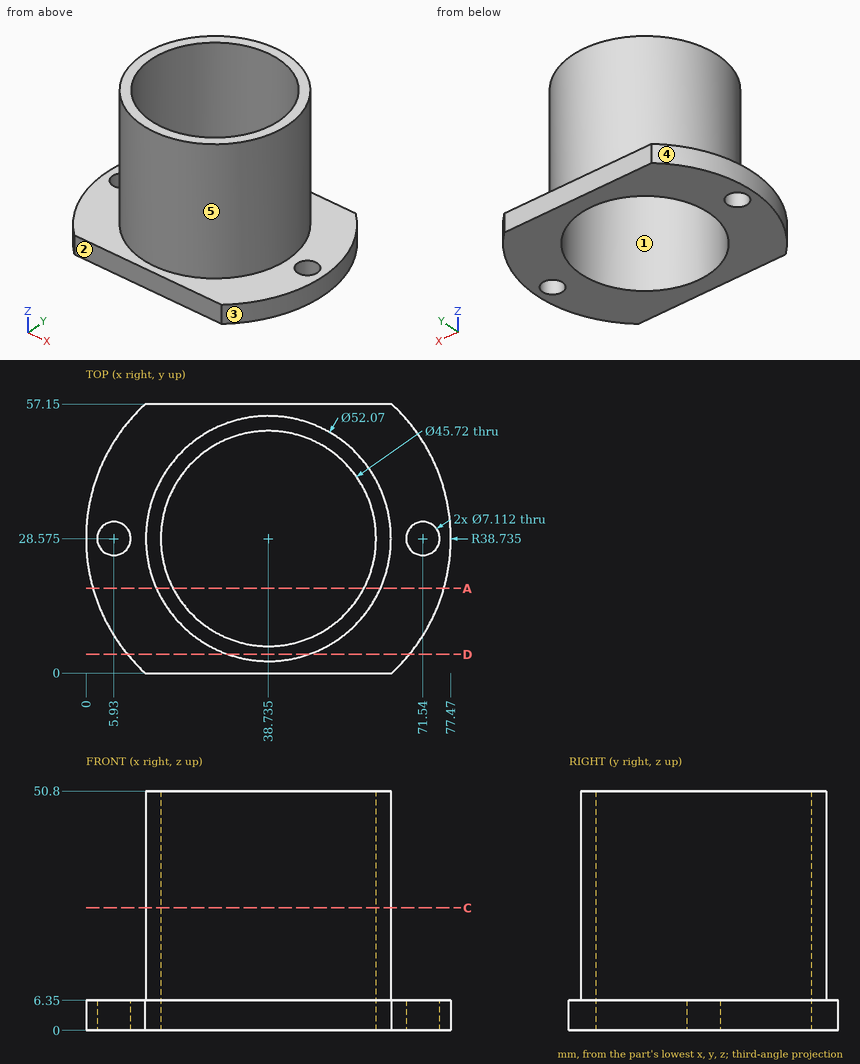
Verification items for this drawing (mm, ordinates from the low corner). A direction names the side the tool comes from. Round coordinates to 2 decimals unless told otherwise and drop trailing zeros. Order: outer loops, then holes, each group sorted by start corner. A loop starts at its lowest first (then second) coordinate and runs counter-clockwise, first axis right, second up. Notation, with made-up numbers: M 37.5,84.5 L 79.5,84.5 A27 cw 79.5,120.5 Z; hole C 59,9 d7. An arc over 180 degrees is marked long. Answer in a Markdown table with one row per item. Add a question column.
Item 1: Draft check along Y on the marked faces 1, 2 and 3. Enter one of: released by +Y, released by -Y, zero draft, split by the parting line, or undercut.
Item 2: Set-up check for the marked faces 4 and 5: record each of +Z, -Z, +X, -X, +Y, -Y from which the full face is reachable in a straight line by a thin tool's end or side.
Item 3: Depth check by flat-ended pin: pin 1 Ø9 at (x, y) = (5.93, 28.58) entering from -Z; pin 2 Ø1.5 at (x, z) = (36, 44) entering from -Y; pin 3 Ø5 at (x, z) = (42.5, 11) entering from +Y; pin 4 Ø1.5 at (x, z) = (41.5, 24.5) entering from +Y. Enter the tip coordinate at first touch or a pass-through.
Item 4: Sectioned sample at C-C, the plane z = 26. Enter the section's corners in (x, y) (3 decimals).
Item 5: Material ranges on L1, parallel to X at y = 28, z = 3; L2, parallel to Y at x = 38, z = 42.5; L3, parallel to X at y = 28.5, z = 47 (1 decimal), recorded low to high. Write a range as [from, to].
Item 6: Sectioned sample at A-A, the plane y = 18. Enter the section's corners in (x, z), plus the area to 3 significant figures.
Item 7: Sectioned sample at D-D, the plane y = 4. Enter the section's corners in (x, z), plus the area to 3 significant figures.
Filled in:
| question | item | result |
|---|---|---|
| 1 | face 1 | undercut |
| 1 | face 2 | released by -Y |
| 1 | face 3 | split by the parting line |
| 2 | face 4 | +Z, -Z, -X |
| 2 | face 5 | +Z |
| 3 | pin 1 | stops at z = 0 |
| 3 | pin 2 | stops at y = 2.62 |
| 3 | pin 3 | stops at y = 54.58 |
| 3 | pin 4 | stops at y = 54.53 |
| 4 | outline | C 38.735,28.575 d52.07; hole C 38.735,28.575 d45.72 |
| 5 | L1 | x = [0, 2.42], [9.44, 15.88], [61.59, 68.03], [75.05, 77.47] |
| 5 | L2 | y = [2.55, 5.73], [51.42, 54.6] |
| 5 | L3 | x = [12.7, 15.9], [61.6, 64.8] |
| 6 | outline | M 1.47,0 L 18.47,0 L 18.47,50.8 L 14.94,50.8 L 14.94,6.35 L 1.47,6.35 Z; M 59,0 L 76,0 L 76,6.35 L 62.53,6.35 L 62.53,50.8 L 59,50.8 Z |
| 6 | area | 529 mm² |
| 7 | outline | M 8.79,0 L 68.68,0 L 68.68,6.35 L 47.33,6.35 L 47.33,50.8 L 30.14,50.8 L 30.14,6.35 L 8.79,6.35 Z |
| 7 | area | 1,140 mm² |
